Work out the finished part from the listing and answer in its coordinate system (mm). Face numbers are marked on the shaded views. A direction names the side the tool comes from. Round coordinates to 2 decimals unless told otherwise and drop trailing zeros. Loops run counter-clockwise (first coordinate to the right, second up) from the corner with the lowest first, then second, coordinate; pieces in that order, holes last.
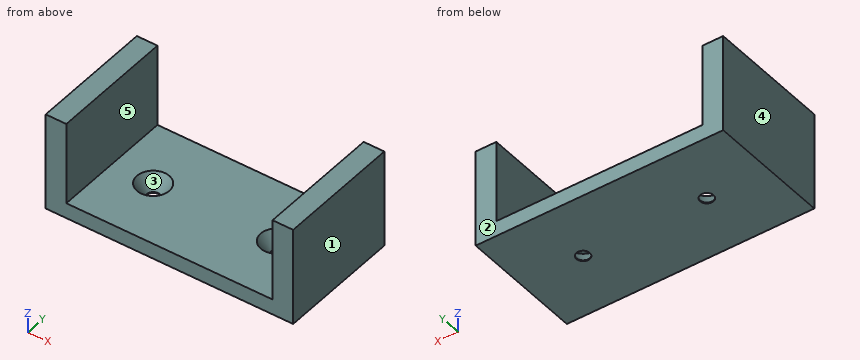
```python
from build123d import *

# Parameters (mm, degrees)
F0_W     = 76.2
F0_H     = 38.1
F0_R     = 2.0574
F1_DEPTH = 4.7625
F2_W     = 6.35
F2_H     = 38.1
F3_DEPTH = 25.4
F4_SIZE2 = 2.921
F4_SIZE  = 4.4704
F5_SIZE2 = 2.921
F5_SIZE  = 4.4704


with BuildPart() as f1:
    # F0 (on Top) → F1 (new body)
    with BuildSketch(Plane.XY):
        Rectangle(F0_W, F0_H)
        with Locations((-19.05, 0)):
            Circle(F0_R, mode=Mode.SUBTRACT)
        with Locations((19.05, 0)):
            Circle(F0_R, mode=Mode.SUBTRACT)
    extrude(amount=F1_DEPTH)

    # F2 (on face) → F3 (join)
    with BuildSketch(Plane.XY.offset(4.7625)):
        with Locations((-34.925, 0)):
            Rectangle(F2_W, F2_H)
        with Locations((34.925, 0)):
            Rectangle(F2_W, F2_H)
    extrude(amount=F3_DEPTH)

    # F4
    f4_edges = [f1.edges().sort_by_distance(p)[0] for p in [
        (-21.1074, 0, 4.7625),
    ]]
    f4_side = f1.faces().sort_by_distance((-21.1074, 0, 2.38125))[0]
    chamfer(f4_edges, length=F4_SIZE, length2=F4_SIZE2, reference=f4_side)

    # F5
    f5_edges = [f1.edges().sort_by_distance(p)[0] for p in [
        (16.9926, 0, 4.7625),
    ]]
    f5_side = f1.faces().sort_by_distance((16.9926, 0, 2.38125))[0]
    chamfer(f5_edges, length=F5_SIZE, length2=F5_SIZE2, reference=f5_side)


solid = f1.part
```
1. Which of the six approach directions +Z, -Z, +X, -X, +Y, -Y give full straight-line access (tool end or side, diameter ignored) to the marked faces 4 and 5?
Answer key:
face 4: +Z, -Z, -X, +Y, -Y
face 5: +Z, +Y, -Y
2. Find section C-C (x = 19.05). Write down the section's boundary in (y, z), then the cut area to 3 significant figures.
Answer key:
outline: (-19.05, 0) - (-2.06, 0) - (-2.06, 0.29) - (-4.98, 4.76) - (-19.05, 4.76) - close; (2.06, 0) - (19.05, 0) - (19.05, 4.76) - (4.98, 4.76) - (2.06, 0.29) - close
area: 149 mm2
3. Find section A-A (z = 10). Write down the section's boundary in (x, y).
Answer key:
outline: (-38.1, -19.05) - (-31.75, -19.05) - (-31.75, 19.05) - (-38.1, 19.05) - close; (31.75, -19.05) - (38.1, -19.05) - (38.1, 19.05) - (31.75, 19.05) - close
4. Consider probe 1 along X at (y, z) = (2, 7); probe 2 along Y at (x, z) = (19.05, 0.25); probe 3 along Z at (x, y) = (-20, -15.5). Determine where each line is inside the solid, lowest interval first.
Answer key:
probe 1: x = -38.1 to -31.75, 31.75 to 38.1
probe 2: y = -19.05 to -2.06, 2.06 to 19.05
probe 3: z = 0 to 4.76
5. Determine the mould class of the marked faces 1, 2 and 3 for opening direction Y: +Y half, -Y half, draft (parallel to the pull), parting line (faces both ways), or undercut.
Answer key:
face 1: draft
face 2: +Y half
face 3: undercut
6. Find section B-B (y = 0). Write down the section's boundary in (x, z), then the cut area to 3 significant figures.
Answer key:
outline: (-38.1, 0) - (-21.11, 0) - (-21.11, 0.29) - (-24.03, 4.76) - (-31.75, 4.76) - (-31.75, 30.16) - (-38.1, 30.16) - close; (-16.99, 0) - (16.99, 0) - (16.99, 0.29) - (14.07, 4.76) - (-14.07, 4.76) - (-16.99, 0.29) - close; (21.11, 0) - (38.1, 0) - (38.1, 30.16) - (31.75, 30.16) - (31.75, 4.76) - (24.03, 4.76) - (21.11, 0.29) - close
area: 620 mm2
7. Given pin 1 (8 mm diameter, centred on x = -10, y = 8, fed in from +Z); pin 2 (3.5 mm diameter, centred on x = 19.05, y = 0, fed in from +Z); pin 3 (6 mm diameter, centred on x = -13, y = 9, fed in from -Z), each flat-ended and moving along its own axis, determine where each tip first touches the part or whether it passes through.
Answer key:
pin 1: stops at z = 4.76
pin 2: passes through
pin 3: stops at z = 0
8. Find section D-D (y = 12.5). Write down the section's boundary in (x, z).
Answer key:
outline: (-38.1, 0) - (38.1, 0) - (38.1, 30.16) - (31.75, 30.16) - (31.75, 4.76) - (-31.75, 4.76) - (-31.75, 30.16) - (-38.1, 30.16) - close
